from build123d import *

# Parameters (mm, degrees)
BOSS_EXTRUDE1_DEPTH = 10.7
SKETCH2_3_W         = 2.36
SKETCH2_3_H         = 1.92
BOSS_EXTRUDE2_DEPTH = 12.7
EXTRUDE_THIN1_START = -9.155
EXTRUDE_THIN1_DEPTH = 18.31
SKETCH5_W           = 23.92
SKETCH5_H           = 0.54
BOSS_EXTRUDE3_DEPTH = 9.88
CUT_EXTRUDE1_DEPTH  = 2
BOSS_EXTRUDE4_DEPTH = 8.7
CUT_EXTRUDE3_DEPTH  = 18.7
BOSS_EXTRUDE5_DEPTH = 8.65
BOSS_EXTRUDE7_DEPTH = 8.65


# Read off the part's stored shape, not the designer's step: Extrude-Thin1
with BuildPart() as part:
    # Sketch2 → Boss-Extrude1 (new, symmetric)
    with BuildSketch(Plane.XY):
        Polygon((12.75, -3.906779661), (12.75, 7.08), (5.116131156, 7.08), (-12.75, 7.08), (-12.75, -3.906779661), (-12.75, -9), (0, -9), (12.75, -9), align=None)
    extrude(amount=BOSS_EXTRUDE1_DEPTH, both=True)

    # Sketch2<3> → Boss-Extrude2 (add, symmetric)
    with BuildSketch(Plane.XY):
        Polygon((-12.75, 7.08), (5.116131156, 7.08), (5.116131156, 9), (0, 9), (-12.12, 9), (-12.75, 9), align=None)
        with Locations((-13.93, 8.04)):
            Rectangle(SKETCH2_3_W, SKETCH2_3_H)
        with Locations((13.93, 8.04)):
            Rectangle(SKETCH2_3_W, SKETCH2_3_H)
        Polygon((5.116131156, 7.08), (12.75, 7.08), (12.75, 9), (12.12, 9), (6.67, 9), (5.116131156, 9), align=None)
    extrude(amount=BOSS_EXTRUDE2_DEPTH, both=True)

    # Extrude-Thin1 outline → Extrude-Thin1 (add)
    with BuildSketch(Plane.XY.offset(EXTRUDE_THIN1_START)):
        with BuildLine():
            add(Edge.make_bspline(
                [(-12.12, 9), (-1.256881612, 9.695668212), (6.67, 15.22)],
                knots=[0, 0, 0, 1, 1, 1], degree=2))
            Line((-12.12, 9), (11.004787045, 9))
            Line((11.004787045, 9), (6.67, 15.22))
        make_face()
    extrude(amount=EXTRUDE_THIN1_DEPTH)

    # Sketch5 → Boss-Extrude3 (add)
    with BuildSketch(Plane.XZ.offset(9)):
        with Locations((0, -0.27)):
            Rectangle(SKETCH5_W, SKETCH5_H)
        with Locations((0, 0.27)):
            Rectangle(SKETCH5_W, SKETCH5_H)
    extrude(amount=BOSS_EXTRUDE3_DEPTH)

    # Sketch6 → Cut-Extrude1 (cut)
    with BuildSketch(Plane(origin=(0, 0, -0.54), x_dir=(-1, 0, 0), z_dir=(0, 0, -1))):
        with BuildLine():
            ThreePointArc((-10.96, -18.88), (-11.667106781, -18.587106781), (-11.96, -17.88))
            Line((-11.96, -17.88), (-11.96, -18.88))
            Line((-11.96, -18.88), (-10.96, -18.88))
        make_face()
        with BuildLine():
            Line((11.96, -18.88), (11.96, -17.88))
            ThreePointArc((11.96, -17.88), (11.667106781, -18.587106781), (10.96, -18.88))
            Line((10.96, -18.88), (11.96, -18.88))
        make_face()
    extrude(amount=-CUT_EXTRUDE1_DEPTH, mode=Mode.SUBTRACT)

    # Sketch7 → Boss-Extrude4 (add)
    with BuildSketch(Plane.XZ.offset(9)):
        Polygon((-11.96, 9.64), (-11.96, 0.54), (-11.01, 0.54), (-11.01, 3.822076599), (-11.01, 9.64), align=None)
        Polygon((-1.16, 3.822076599), (-1.16, 0.54), (-0.21, 0.54), (-0.21, 9.64), (-1.16, 9.64), align=None)
        Polygon((-0.21, -0.54), (-1.16, -0.54), (-1.16, -5.923650712), (-1.16, -9.64), (-0.21, -9.64), align=None)
        Polygon((-11.01, -0.54), (-11.96, -0.54), (-11.96, -9.64), (-11.01, -9.64), (-11.01, -5.923650712), align=None)
    extrude(amount=BOSS_EXTRUDE4_DEPTH)

    # Sketch8 → Cut-Extrude3 (cut)
    with BuildSketch(Plane.ZY.offset(11.96)):
        with BuildLine():
            Line((-8.24, -9), (-9.64, -9))
            Line((-9.64, -9), (-9.64, -17.7))
            Line((-9.64, -17.7), (-7.94, -17.7))
            ThreePointArc((-7.94, -17.7), (-8.152132034, -17.612132034), (-8.24, -17.4))
            Line((-8.24, -17.4), (-8.24, -9))
        make_face()
        with BuildLine():
            Line((-0.54, -9), (-1.94, -9))
            Line((-1.94, -9), (-1.94, -17.4))
            ThreePointArc((-1.94, -17.4), (-2.027867966, -17.612132034), (-2.24, -17.7))
            Line((-2.24, -17.7), (-0.54, -17.7))
            Line((-0.54, -17.7), (-0.54, -9))
        make_face()
        with BuildLine():
            ThreePointArc((-4.33865298, -13.35), (-5.09, -12.59865298), (-5.84134702, -13.35))
            Line((-5.84134702, -13.35), (-5.231421356, -13.959925664))
            ThreePointArc((-5.231421356, -13.959925664), (-5.09, -14.018504308), (-4.948578644, -13.959925664))
            Line((-4.948578644, -13.959925664), (-4.33865298, -13.35))
        make_face()
        with BuildLine():
            Line((1.94, -9), (0.54, -9))
            Line((0.54, -9), (0.54, -17.7))
            Line((0.54, -17.7), (2.24, -17.7))
            ThreePointArc((2.24, -17.7), (2.027867966, -17.612132034), (1.94, -17.4))
            Line((1.94, -17.4), (1.94, -9))
        make_face()
        with BuildLine():
            Line((9.64, -9), (8.24, -9))
            Line((8.24, -9), (8.24, -17.4))
            ThreePointArc((8.24, -17.4), (8.152132034, -17.612132034), (7.94, -17.7))
            Line((7.94, -17.7), (9.64, -17.7))
            Line((9.64, -17.7), (9.64, -9))
        make_face()
        with BuildLine():
            ThreePointArc((5.84134702, -13.35), (5.09, -12.59865298), (4.33865298, -13.35))
            Line((4.33865298, -13.35), (4.948578644, -13.959925664))
            ThreePointArc((4.948578644, -13.959925664), (5.09, -14.018504308), (5.231421356, -13.959925664))
            Line((5.231421356, -13.959925664), (5.84134702, -13.35))
        make_face()
    extrude(amount=-CUT_EXTRUDE3_DEPTH, mode=Mode.SUBTRACT)

    # Sketch2<13> → Boss-Extrude5 (add, symmetric)
    with BuildSketch(Plane.XY):
        Polygon((14.248489171, 6.709143574), (15.11, 3.02), (12.75, -9), (12.75, -3.906779661), (14.11, 3.02), (13.248489171, 6.709143574), align=None)
    extrude(amount=BOSS_EXTRUDE5_DEPTH, both=True)

    # Sketch2<16> → Boss-Extrude7 (add, symmetric)
    with BuildSketch(Plane.XY):
        Polygon((-12.75, -3.906779661), (-12.75, -9), (-15.11, 3.02), (-14.248489171, 6.709143574), (-13.248489171, 6.709143574), (-14.11, 3.02), align=None)
    extrude(amount=BOSS_EXTRUDE7_DEPTH, both=True)


solid = part.part
Can you work these out from the model? Positions are in its coordinate system, mm. A direction names the side the tool comes from. Coordinates: 2 decimals unless noted, no trailing zeros. Loops run counter-clockwise (first coordinate to the right, second up) from the corner with the lowest first, then second, coordinate; pieces in that order, holes last. Notation, with made-up numbers: (31, 2) - (87, 2) arc R23 ccw to (87, 41) - close; hole circle Ø1 at (19, 81). An arc over 180 degrees is marked (long way). Answer as a JSON object with one key per item and string values. Group by question number.
Item 1: If we section it at A-A (x = 10.5): List the corners of the cut face in (y, z) for me (3 decimals).
Item 2: On a 3-axis mill with a long thin cutter (end or side, diameter ignored), from which of +Z, -Z, +X, -X, +Y, -Y can I reach the whole of each face in a straight line? I mean faces 4 (the face through (2, 11, 9.155)), 5 (the face through (2, 11, -9.155)), 6 (the face through (0, 9, -11)), 7 (the face through (-11.5, -17.7, 5.1)), 8 (the face through (-11.01, -14.3, -5.1)). Say none if no direction works.
Item 3: If I drill on L1, parallel to X at y = 3, z = 3; L2, parallel to X at y = -10.5, z = -7.25; L3, parallel to X at y = 1.5, z = 2, over which ranges is the centre line in solid material (lowest first)? Write a range as from..to.
Item 4: If we mould it in two halves opening along X, with no side actions, what happens to faces 1 (the face through (-11.96, -14.3, 5.1)), 2 (the face through (-12.75, 1, 0)), 3 (the face through (14, 0, -8.65))? For each: released by +X, released by -X, zero draft, split by the parting line, or undercut.
Item 5: For pin 1 (0.8 mm diameter, centred on x = -11.5, y = -14.5, fed in from +Z); pin 2 (3 mm diameter, centred on y = -15.5, z = -4, fed in from +X); pin 3 (5 mm diameter, centred on x = -4.5, y = 12, fed in from -Z) (3 decimals), each with a flat end and sliding along its axis, tell me the tip position at first contact or that it passes through.
Item 6: If we section it at B-B (y = -4.5): List the corners of the cut face in (x, z) for me.
Returned:
{
 "1": {"outline": "(-18.88, -0.54) - (-9, -0.54) - (-9, -10.7) - (7.08, -10.7) - (7.08, -12.7) - (9, -12.7) - (9, -9.155) - (9.724, -9.155) - (9.724, 9.155) - (9, 9.155) - (9, 12.7) - (7.08, 12.7) - (7.08, 10.7) - (-9, 10.7) - (-9, 0.54) - (-18.88, 0.54) - close"},
 "2": {"face 4": "+Z, +X, -X, +Y", "face 5": "-Z, +X, -X, +Y", "face 6": "+Y", "face 7": "+Z, +X, -X, -Y", "face 8": "-Z, -Y"},
 "3": {"L1": "x = -15.11..-14.11, -12.75..12.75, 14.11..15.11", "L2": "x = -11.96..-11.01, -1.16..-0.21", "L3": "x = -14.81..-13.81, -12.75..12.75, 13.81..14.81"},
 "4": {"face 1": "released by -X", "face 2": "undercut", "face 3": "zero draft"},
 "5": {"pin 1": "stops at z = 8.24", "pin 2": "stops at x = -0.21", "pin 3": "stops at z = -9.155"},
 "6": {"outline": "(-13.63, -8.65) - (-12.75, -8.65) - (-12.75, -10.7) - (12.75, -10.7) - (12.75, -8.65) - (13.63, -8.65) - (13.63, 8.65) - (12.75, 8.65) - (12.75, 10.7) - (-12.75, 10.7) - (-12.75, 8.65) - (-13.63, 8.65) - close"}
}
